Input: part model. Units: mm. Frame: model coordinates. A direction names the side the tool comes from. Coordinates: 2 decimals unless noted, no trailing zeros. Loops run counter-clockwise (first coordinate to the right, second up) from the corner with the lowest first, then second, coordinate; pieces in that order, holes last. Notation, with made-up numbers: (86.5, 74.5) -> (134.5, 74.5) arc R35 cw to (134.5, 110.5) -> close; hole circle Ø8 at (-36.5, 65.5). An arc over 180 degrees is marked (long way). Put each result on its own line as item: value. Start each with the question number.
1) Pull-direction query (Y, two-part tool) for faces 1 (the flat face through (-1, 0, 0)), 2 (the flat face through (-1, 6, 64)), 3 (the flat face through (-37.5, 0, 67)), 4 (the flat face through (37.5, 0, 67)); classes: pulls with the +Y half, pulls with the -Y half, needs draft (parallel to the pull), parting line crosses it, or undercut.
2) Material intervals for L1, parallel to Y at x = -4.5, z = 88.5; L2, parallel to X at y = -1.5, z = 8; L3, parallel to Z at x = 0, y = 4.3, sorted ascending.
3) Cut plane B-B (z = 22). Return the cut outline in (x, y).
4) Set-up query: faces 5 (the cylindrical face through (-0.535, -4.859, 127.582)), 6 (the flat face through (-1, 3.75, 67)). Return all of +Z, -Z, +X, -X, +Y, -Y with unobstructed straight access to the full face (end or side cutting, diameter ignored); none if empty.
5) Cut plane C-C (x = -15). Return the cut outline in (y, z), plus the area to 4 significant figures.
6) Contact query for flat-ended pins moving along their axis: P1, Ø2, axis at x = 12.5, y = -1, coming from the +Z side; P2, Ø1, axis at y = -3.5, z = 108, coming from the +X side. Output: stop coordinate, or through.
7) Cut plane A-A (x = 0). Return the cut outline in (y, z), plus the area to 3 significant figures.
from build123d import *

# Parameters (mm, degrees)
F0_W          = 84
F0_H          = 12
F1_DEPTH      = 130
F3_W          = 75
F3_H          = 7.5
F4_DEPTH      = 127
F5_R          = 5
F6_R          = 4.1062425904
F7_DEPTH      = 6.001
F7_DEPTH_BACK = 25


with BuildPart() as f1:
    # F0 (on Top) → F1 (new body)
    with BuildSketch(Plane.XY):
        Rectangle(F0_W, F0_H)
    extrude(amount=F1_DEPTH)

    # F3 (on offset) → F4 (cut)
    with BuildSketch(Plane.XY.offset(130)):
        Rectangle(F3_W, F3_H)
    extrude(amount=-F4_DEPTH, mode=Mode.SUBTRACT)

    # F5
    f5_edges = [f1.edges().sort_by_distance(p)[0] for p in [
        (42, -6, 65),
        (42, 6, 65),
        (-42, 6, 65),
        (-42, -6, 65),
    ]]
    fillet(f5_edges, radius=F5_R)

    # F6 (on Front) → F7 (cut, two sides)
    with BuildSketch(Plane.XZ) as f7_sk:
        with Locations((0, 123.5107928514)):
            Circle(F6_R)
    extrude(amount=-F7_DEPTH, mode=Mode.SUBTRACT)
    extrude(f7_sk.sketch, amount=F7_DEPTH_BACK, mode=Mode.SUBTRACT)


solid = f1.part
Results found:
1. face 1: needs draft
1. face 2: pulls with the +Y half
1. face 3: undercut
1. face 4: undercut
2. L1: y = -6 to -3.75, 3.75 to 6
2. L2: x = -41.97 to -37.5, 37.5 to 41.97
2. L3: z = 0 to 119.4, 127.62 to 130
3. outline: (-42, -1) arc R5 ccw to (-37, -6) -> (37, -6) arc R5 ccw to (42, -1) -> (42, 1) arc R5 ccw to (37, 6) -> (-37, 6) arc R5 ccw to (-42, 1) -> close; hole (-37.5, -3.75) -> (37.5, -3.75) -> (37.5, 3.75) -> (-37.5, 3.75) -> close
4. face 5: +Y, -Y
4. face 6: +Z
5. outline: (-6, 0) -> (6, 0) -> (6, 130) -> (3.75, 130) -> (3.75, 3) -> (-3.75, 3) -> (-3.75, 130) -> (-6, 130) -> close
5. area: 607.5 mm2
6. P1: stops at z = 3
6. P2: stops at x = 41.58
7. outline: (-6, 0) -> (6, 0) -> (6, 119.4) -> (3.75, 119.4) -> (3.75, 3) -> (-3.75, 3) -> (-3.75, 119.4) -> (-6, 119.4) -> close; (-6, 127.62) -> (-3.75, 127.62) -> (-3.75, 130) -> (-6, 130) -> close; (3.75, 127.62) -> (6, 127.62) -> (6, 130) -> (3.75, 130) -> close
7. area: 571 mm2
